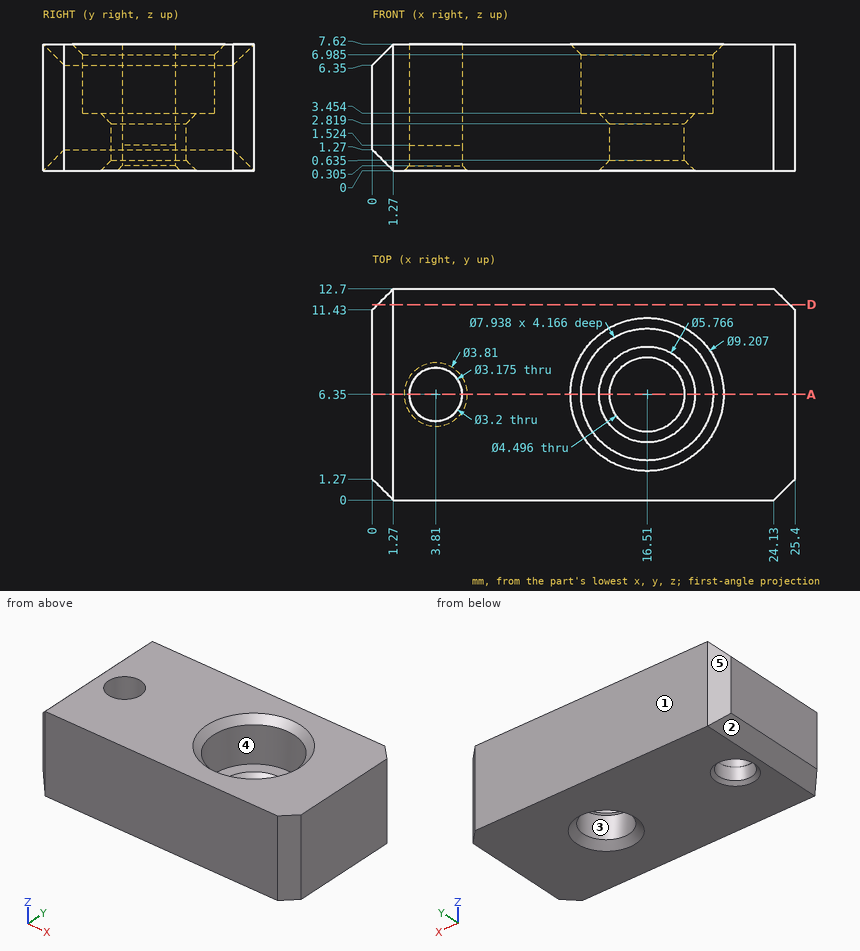
For this review, use the dimensioned drawing (mm, ordinates from the lowest corner) and the shaded views. A direction names the side the tool comes from. Round coordinates to 2 decimals unless told otherwise and drop trailing zeros. Write each loop counter-clockwise with the first axis right and the second up, starting at its lowest first coordinate (ties: lowest second). Pieces come first, ordered by that corner, then holes. Notation, with made-up numbers: (5, 81) - (57, 81) arc R19 cw to (57, 118) - close; hole circle Ø1 at (7, 3.25). An arc over 180 degrees is marked (long way). Answer as CSV lines item,"result". Start each with the question number.
(1) For pin 1 Ø7 at (x, y) = (16.51, 6.35) entering from +Z; pin 2 Ø5 at (x, y) = (16.51, 6.35) entering from -Z, all flat-tipped, find the tip position at first contact; note any pin that passes through.
(2) We need section A-A on y = 6.35. Give the number of separate pieces and of enclosed holes in the cut face, plus the area to 3 significant figures.
(3) For the marked faces 4 and 5, list the 3-axis set-ups (+Z, -Z, +X, -X, +Y, -Y) from which the entire face can be reached by the end or side of a thin tool; tool diameter is ignored.
(4) To check wall thickness, follow line 1 (X direction, y = 6.35, z = 2.45); line 2 (X direction, y = 6.35, z = 6); line 3 (Y direction, x = 16.51, z = 2.1). State the ranges of each line that lie inside material, in increasing order.
(5) We need section D-D on y = 11.75. State the section outline as (x, z) points.
(6) Draft analysis for pull direction Y (two halves, no side actions). For the marked faces 1, 2 and 3, state which applies: pulls with the +Y half, pulls with the -Y half, needs draft (parallel to the pull), parting line crosses it, or undercut.
Worked answers:
1,pin 1,"z = 3.45"
1,pin 2,"z = 0.38"
2,separate pieces,"3"
2,enclosed holes,"0"
2,area,"118 mm²"
3,face 4,"+Z"
3,face 5,"+Z, -Z, -X, +Y"
4,line 1,"0 to 2.22, 5.4 to 14.26, 18.76 to 25.4"
4,line 2,"0 to 2.22, 5.4 to 12.54, 20.48 to 25.4"
4,line 3,"0 to 4.1, 8.6 to 12.7"
5,outline,"(0.32, 0.95) - (1.27, 0) - (25.08, 0) - (25.08, 7.62) - (1.27, 7.62) - (0.32, 6.67) - close"
6,face 1,"pulls with the +Y half"
6,face 2,"needs draft"
6,face 3,"undercut"
